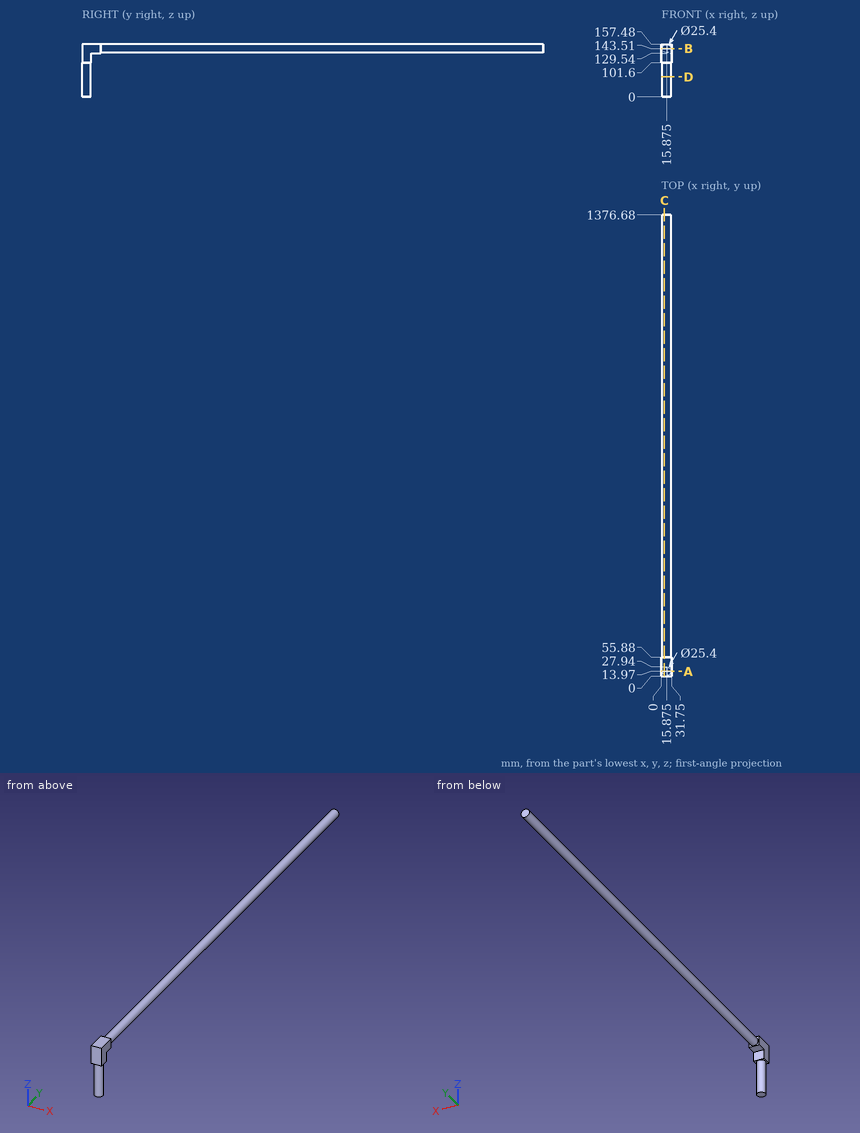
Drawing for the job (mm, zero at the part's lowest x, y, z). Round coordinates to 2 decimals unless told otherwise and drop trailing zeros. Order: outer loops, then holes, each group sorted by start corner. A loop starts at its lowest first (then second) coordinate and runs counter-clockwise, first axis right, second up.
Item 1: Saw through at C-C on x = 9. Write the cut outline in (y, z).
Item 2: Saw through at A-A on y = 13.97. Write the cut outline in (x, z) (3 decimals), then the cut area to 3 significant figures.
Item 3: Saw through at B-B on z = 143.51. Write the cut outline in (x, y) (3 decimals).
Item 4: Saw through at D-D on z = 59.5. Write the cut outline in (x, y) (3 decimals), then the cut area to 3 significant figures.
Item 5: Pin check, flat tips, straight feed: pin 1 (5 mm diameter, centred on x = 18.5, y = 283, fed in from -Z); pin 2 (2 mm diameter, centred on x = 18, y = 863, fed in from +Z); pin 3 (4 mm diameter, centred on x = 20.5, y = 928, fed in from +Z). Stop position of each tip, or through.
Item 6: Probe line 1 along Z through (x, y) = (14, 947); line 2 along Z through (x, y) = (17.5, 1189); line 3 along Y through (x, z) = (16.5, 114). List the from-to ranges inside material, lowest first.
Reported:
1. outline: (0, 101.6) - (3.29, 101.6) - (3.29, 0) - (24.65, 0) - (24.65, 101.6) - (27.94, 101.6) - (27.94, 129.54) - (55.88, 129.54) - (55.88, 132.83) - (1376.68, 132.83) - (1376.68, 154.19) - (55.88, 154.19) - (55.88, 157.48) - (0, 157.48) - close
2. outline: (0, 101.6) - (3.175, 101.6) - (3.175, 0) - (28.575, 0) - (28.575, 101.6) - (31.75, 101.6) - (31.75, 157.48) - (0, 157.48) - close
2. area: 4,350 mm2
3. outline: (0, 0) - (31.75, 0) - (31.75, 55.88) - (28.575, 55.88) - (28.575, 1376.68) - (3.175, 1376.68) - (3.175, 55.88) - (0, 55.88) - close
4. outline: circle Ø25.4 at (15.875, 13.97)
4. area: 507 mm2
5. pin 1: stops at z = 130.81
5. pin 2: stops at z = 156.16
5. pin 3: stops at z = 155.94
6. line 1: z = 130.95 to 156.07
6. line 2: z = 130.91 to 156.11
6. line 3: y = 0 to 27.94
